Design review of the part built by this model. Coordinates are the model's own, in mm. Face numbers are marked on the shaded views. A direction names the side the tool comes from. Give positions to 0.01 mm unless a question says otherwise; leave off trailing zeros. Order: outer loops, then holes, each group sorted by start corner. A loop starts at its lowest first (then second) coordinate and runs counter-clockwise, first axis right, second up. Notation, with made-up numbers: M 25.5,24 L 36.5,24 A24 ccw 36.5,46 Z; hole C -13,75 d4. An arc over 180 degrees is marked long. Answer as a JSON object with one key per item and string values.
from build123d import *

# Parameters (mm, degrees)
F0_W     = 158.276036
F0_H     = 135.355964
F1_DEPTH = 66.04
F2_R     = 27.36159
F3_DEPTH = 76.962
F4_W     = 65.755699
F4_H     = 20.332886
F5_DEPTH = 178.308


with BuildPart() as f1:
    # F0 (on Top) → F1 (new body)
    with BuildSketch(Plane.XY):
        with Locations((-79.138018, -67.677982)):
            Rectangle(F0_W, F0_H)
    extrude(amount=F1_DEPTH)

    # F2 (on face) → F3 (join)
    with BuildSketch(Plane.XY.offset(66.04)):
        with Locations((-110.367209, -68.513423)):
            Circle(F2_R)
    extrude(amount=F3_DEPTH)

    # F4 (on face) → F5 (cut)
    with BuildSketch(Plane.XZ.offset(135.355964)):
        with Locations((-74.039189, 30.590639)):
            Rectangle(F4_W, F4_H)
    extrude(amount=-F5_DEPTH, mode=Mode.SUBTRACT)


solid = f1.part
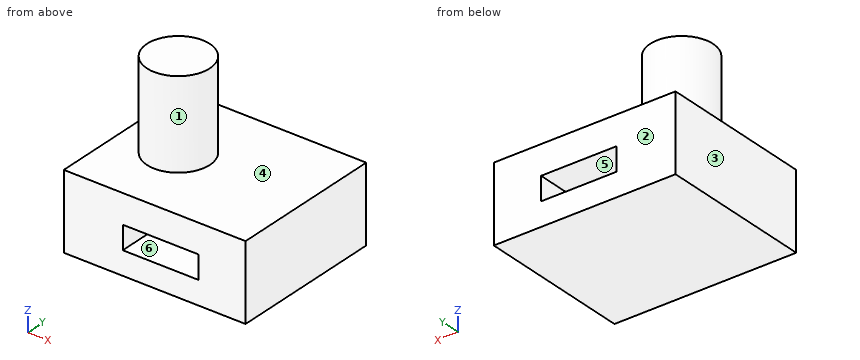
(1) We need section B-B (y = -82.5). Write out the cut boundary in (x, z), plus the area to 3 significant figures.
Checked values:
{"outline": "M -158.28,0 L 0,0 L 0,66.04 L -86.85,66.04 L -86.85,143 L -133.88,143 L -133.88,66.04 L -158.28,66.04 Z; hole M -106.92,20.42 L -41.16,20.42 L -41.16,40.76 L -106.92,40.76 Z", "area": "12,700 mm^2"}
(2) Draft analysis for pull direction X (two halves, no side actions). For the marked faces 3, 4, 5 and 6, state which applies: +X half, -X half, draft (parallel to the pull), parting line (faces both ways), or undercut.
Checked values:
{"face 3": "-X half", "face 4": "draft", "face 5": "undercut", "face 6": "undercut"}
(3) To check wall thickness, follow L1, parallel to Z at x = -88, y = -80.5; L2, parallel to Z at x = -74, y = -122; L3, parallel to X at y = -54.5, z = 40. State the ranges of each line that lie inside material, in increasing order. Write a range as from..to.
Checked values:
{"L1": "z = 0..20.42, 40.76..143", "L2": "z = 0..20.42, 40.76..66.04", "L3": "x = -158.28..-106.92, -41.16..0"}
(4) Insertion check: pin 1 (3 mm diameter, centred on x = -56.5, y = -24.5, fed in from +Z); pin 2 (1 mm diameter, centred on y = -66, z = 103, fed in from +X); pin 3 (12 mm diameter, centred on x = -106, z = 123, fed in from -Y) (3 decimals). Each pin has a flat end and moves straight along its axis. Give the tip position at first contact, or say it passes through.
Checked values:
{"pin 1": "stops at z = 66.04", "pin 2": "stops at x = -83.08", "pin 3": "stops at y = -95.875"}
(5) Tool access review of the marked faces 1 and 2: name each direction out of +Z, -Z, +X, -X, +Y, -Y from which nothing blocks a thin tool from reaching the whole face with its end or side.
Checked values:
{"face 1": "+Z", "face 2": "+Z, -Z, +X, -X, +Y"}
(6) We need section C-C (x = -117.5). Write out the cut boundary in (y, z), plus the area to 3 significant figures.
Checked values:
{"outline": "M -135.36,0 L 0,0 L 0,66.04 L -42.1,66.04 L -42.1,143 L -94.93,143 L -94.93,66.04 L -135.36,66.04 Z", "area": "13,000 mm^2"}
(7) We need section A-A (x = -77). Write out the cut boundary in (y, z).
Checked values:
{"outline": "M -135.36,0 L 0,0 L 0,20.42 L -135.36,20.42 Z; M -135.36,40.76 L 0,40.76 L 0,66.04 L -135.36,66.04 Z"}
(8) We need section D-D (y = -44.5). Write out the cut boundary in (x, z).
Checked values:
{"outline": "M -158.28,0 L 0,0 L 0,66.04 L -97.25,66.04 L -97.25,143 L -123.48,143 L -123.48,66.04 L -158.28,66.04 Z; hole M -106.92,20.42 L -41.16,20.42 L -41.16,40.76 L -106.92,40.76 Z"}
